Can you work these out from the model? Positions are in its coordinate system, mm. A direction names the side the tool comes from. Coordinates: 2 decimals unless noted, no trailing zeros. Order: outer loops, then holes, each group sorted by start corner. A loop starts at its lowest first (then second) coordinate and runs counter-clockwise, first axis right, second up. Notation, with made-up numbers: (12, -29) -> (50, -29) arc R19 cw to (50, 6) -> close; hole circle Ø1 at (79.5, 42). An arc over 180 degrees is marked (long way). Use a Markdown table: item, result. Add a question column.
1. We'd pull the mould along X, two halves only. Please class faces 1 (the flat face through (-12, -19, 107)), 2 (the flat face through (-88, -4, 116.674)): pulls with the +X half, pulls with the -X half, needs draft (parallel to the pull), parting line crosses it, or undercut.
2. Suppose I cut it at D-D, the plane y = -12.75. List the corners of the cut face in (x, z) for me, then the cut area to 3 significant figures.
3. Suppose I cut it at B-B, the plane z = 191. List the corners of the cut face in (x, y) for me, then the cut area to 3 significant figures.
4. If I drill on line 1 along X through (y, z) = (-5.5, 20); line 2 along Z through (x, y) = (27.5, -3); line 3 along Z through (x, y) = (-109, -3.25), over which ranges is the centre line in solid material (lowest first)? Write a range as from..to.
5. For faces 3 (the flat face through (98, -4, 146.674)), 4 (the cylindrical face through (-21.98, -13.58, 105.39)), which set-ups out of +Z, -Z, +X, -X, +Y, -Y let a thin tool reach every point of the face, with its end or its side?
6. Suppose I cut it at C-C, the plane x = -114.5. List the corners of the cut face in (y, z) for me.
7. Suppose I cut it at A-A, the plane x = -81.5. List the corners of the cut face in (y, z) for me.
```python
from build123d import *

# Parameters (mm, degrees)
F0_W     = 300
F0_H     = 400
F1_DEPTH = 19
F2_R     = 37
F2_R_2   = 92
F3_DEPTH = 19
F5_DEPTH = 8


with BuildPart() as f1:
    # F0 (on Front) → F1 (new body)
    with BuildSketch(Plane.XZ):
        with Locations((-10.006191, 59.673727)):
            Rectangle(F0_W, F0_H)
    extrude(amount=F1_DEPTH)

    # F2 (on face) → F3 (cut)
    with BuildSketch(Plane.XZ.offset(19)):
        with Locations((-10.006191, 172.673727)):
            Circle(F2_R)
        with Locations((-10.006191, 14.173727)):
            Circle(F2_R_2)
    extrude(amount=-F3_DEPTH, mode=Mode.SUBTRACT)

    # F4 (on face) → F5 (cut)
    with BuildSketch(Plane(origin=(0, 0, 0), x_dir=(-1, 0, 0), z_dir=(0, 1, 0))):
        Polygon((119.506191, -88.326273), (-129.493809, -88.326273), (-129.493809, -118.326273), (149.506191, -118.326273), (149.506191, 146.673727), (87.006191, 146.673727), (87.006191, 179.673727), (149.506191, 179.673727), (149.506191, 249.673727), (-129.493809, 249.673727), (-129.493809, 179.673727), (-66.993809, 179.673727), (-66.993809, 146.673727), (-129.493809, 146.673727), (-129.493809, -78.326273), (102.506191, -78.326273), (102.506191, 106.673727), (-82.493809, 106.673727), (-82.493809, -48.326273), (-99.493809, -48.326273), (-99.493809, 116.673727), (-36.993809, 116.673727), (-36.993809, 209.673727), (-99.493809, 209.673727), (-99.493809, 219.673727), (119.506191, 219.673727), (119.506191, 209.673727), (57.006191, 209.673727), (57.006191, 116.673727), (119.506191, 116.673727), align=None)
    extrude(amount=-F5_DEPTH, mode=Mode.SUBTRACT)


solid = f1.part
```
Worked out:
| question | item | result |
|---|---|---|
| 1 | face 1 | needs draft |
| 1 | face 2 | undercut |
| 2 | outline | (-160.01, -140.33) -> (139.99, -140.33) -> (139.99, 259.67) -> (-160.01, 259.67) -> close; hole circle Ø184 at (-10.01, 14.17); hole circle Ø74 at (-10.01, 172.67) |
| 2 | area | 89,100 mm² |
| 3 | outline | (-160.01, -19) -> (-42.15, -19) -> (-42.15, 0) -> (-57.01, 0) -> (-57.01, -8) -> (-149.51, -8) -> (-149.51, 0) -> (-160.01, 0) -> close; (22.14, -19) -> (139.99, -19) -> (139.99, 0) -> (129.49, 0) -> (129.49, -8) -> (36.99, -8) -> (36.99, 0) -> (22.14, 0) -> close |
| 3 | area | 3,000 mm² |
| 4 | line 1 | x = -160.01..-149.51, -119.51..-102.51, 82.49..99.49, 129.49..139.99 |
| 4 | line 2 | z = -140.33..-118.33, -88.33..-78.33, 106.67..219.67, 249.67..259.67 |
| 4 | line 3 | z = -140.33..-118.33, -88.33..116.67, 146.67..179.67, 209.67..219.67, 249.67..259.67 |
| 5 | face 3 | +Y |
| 5 | face 4 | +Y, -Y |
| 6 | outline | (-19, -140.33) -> (0, -140.33) -> (0, -118.33) -> (-8, -118.33) -> (-8, -88.33) -> (0, -88.33) -> (0, 116.67) -> (-8, 116.67) -> (-8, 146.67) -> (0, 146.67) -> (0, 179.67) -> (-8, 179.67) -> (-8, 209.67) -> (0, 209.67) -> (0, 219.67) -> (-8, 219.67) -> (-8, 249.67) -> (0, 249.67) -> (0, 259.67) -> (-19, 259.67) -> close |
| 7 | outline | (-19, -140.33) -> (0, -140.33) -> (0, -118.33) -> (-8, -118.33) -> (-8, -88.33) -> (0, -88.33) -> (0, -78.33) -> (-8, -78.33) -> (-8, -43.73) -> (-19, -43.73) -> close; (-19, 72.08) -> (-8, 72.08) -> (-8, 106.67) -> (0, 106.67) -> (0, 116.67) -> (-8, 116.67) -> (-8, 209.67) -> (0, 209.67) -> (0, 219.67) -> (-8, 219.67) -> (-8, 249.67) -> (0, 249.67) -> (0, 259.67) -> (-19, 259.67) -> close |
